```python
from build123d import *

# Parameters (mm, degrees)
SKETCH1_R           = 20
SKETCH1_R_2         = 2.75
BOSS_EXTRUDE1_DEPTH = 5
FILLET1_R           = 20


with BuildPart() as part:
    # Sketch1 → Boss-Extrude1 (new body)
    with BuildSketch(Plane.XY):
        Polygon((25, 0), (-25, 0), (-50, 145), (50, 145), align=None)
        with Locations((0, 100)):
            Circle(SKETCH1_R, mode=Mode.SUBTRACT)
        with Locations((-18.384776311, 118.384776311)):
            Circle(SKETCH1_R_2, mode=Mode.SUBTRACT)
        with Locations((-18.384776311, 81.615223689)):
            Circle(SKETCH1_R_2, mode=Mode.SUBTRACT)
        with Locations((18.384776311, 81.615223689)):
            Circle(SKETCH1_R_2, mode=Mode.SUBTRACT)
        with Locations((18.384776311, 118.384776311)):
            Circle(SKETCH1_R_2, mode=Mode.SUBTRACT)
    extrude(amount=BOSS_EXTRUDE1_DEPTH)

    # Fillet1
    fillet1_edges = [part.edges().sort_by_distance(p)[0] for p in [
        (-50, 145, 2.5),
        (50, 145, 2.5),
    ]]
    fillet(fillet1_edges, radius=FILLET1_R)


solid = part.part
```
Source: CAD feature listing. Evaluate the final solid. Frame: model axes, mm. Give positions to 0.01 mm unless a question says otherwise; leave off trailing zeros. Write each loop counter-clockwise with the first axis right and the second up, starting at its lowest first coordinate (ties: lowest second). Pieces come first, ordered by that corner, then holes.
1. First-contact query: pin 1 (3.5 mm diameter, centred on x = -18.38, y = 81.62, fed in from +Z); pin 2 (2 mm diameter, centred on y = 63, z = 1, fed in from -X); pin 3 (1.5 mm diameter, centred on y = 114.5, z = 2, fed in from +X). Flat tips, straight axial feed; report the tip coordinate or a pass-through.
2. Pull-direction query (X, two-part tool) for faces 1 (the face through (41.709, 137.697, 2.535)), 2 (the face through (1, 74, 0)), 3 (the face through (-18.98, 78.93, 2.46)), 4 (the face through (-41.709, 137.697, 2.535)); classes: +X half, -X half, draft (parallel to the pull), parting line (faces both ways), or undercut.
3. Section query A-A (x = 0). Return the cut outline in (y, z).
4. Section query D-D (x = 30.5). Return the cut outline in (y, z), then the cut area to 3 significant figures.
5. Material intervals for line 1 along Y through (x, z) = (16, 2.2); line 2 along X through (y, z) = (96.5, 0.55); line 3 along Y through (x, z) = (13, 1.4), sorted ascending.
6. Section query C-C (y = 100). Return the cut outline in (x, z), then the cut area to 3 significant figures.
7. Section query B-B (z = 1.15). Return the cut outline in (x, y).
Output values:
1. pin 1: passes through
1. pin 2: stops at x = -36.03
1. pin 3: stops at x = 44.87
2. face 1: +X half
2. face 2: draft
2. face 3: undercut
2. face 4: -X half
3. outline: (0, 0) - (80, 0) - (80, 5) - (0, 5) - close; (120, 0) - (145, 0) - (145, 5) - (120, 5) - close
4. outline: (31.9, 0) - (144.54, 0) - (144.54, 5) - (31.9, 5) - close
4. area: 563 mm2
5. line 1: y = 0 to 80.25, 82.98 to 88, 112 to 117.02, 119.75 to 145
5. line 2: x = -41.64 to -19.69, 19.69 to 41.64
5. line 3: y = 0 to 84.8, 115.2 to 145
6. outline: (-42.24, 0) - (-20, 0) - (-20, 5) - (-42.24, 5) - close; (20, 0) - (42.24, 0) - (42.24, 5) - (20, 5) - close
6. area: 222 mm2
7. outline: (-45.97, 121.6) - (-25, 0) - (25, 0) - (45.97, 121.6) arc R20 ccw to (26.26, 145) - (-26.26, 145) arc R20 ccw to start; hole circle Ø5.5 at (-18.38, 81.62); hole circle Ø5.5 at (-18.38, 118.38); hole circle Ø40 at (0, 100); hole circle Ø5.5 at (18.38, 81.62); hole circle Ø5.5 at (18.38, 118.38)
